For this review, take the finished solid that the model builds, in its own axes (mm). A direction names the side the tool comes from. Give positions to 0.01 mm unless a question says otherwise; leave off trailing zeros. Loops run counter-clockwise (first coordinate to the right, second up) from the corner with the lowest first, then second, coordinate; pieces in that order, holes last.
```python
from build123d import *

# Parameters (mm, degrees)
SKETCH001_W  = 85.039572
SKETCH001_H  = 4.2
POCKET_DEPTH = 20


with BuildPart() as part:
    # CopyCopySketch004 → Revolution (revolve)
    with BuildSketch(Plane.XY):
        with BuildLine():
            Line((-94.301748, 7.336546), (-74.200088, 11.003772))
            ThreePointArc((-66.09792, 11.907295), (-70.164685, 11.596147), (-74.200088, 11.003772))
            Line((-66.09792, 11.907295), (-63.874209, 12))
            Line((-63.874209, 12), (-63.874209, 0))
            Line((-63.874209, 0), (-101.154209, 0))
            ThreePointArc((-94.301748, 7.336546), (-98.941677, 4.801888), (-101.154209, 0))
        make_face()
    revolve(axis=Axis((0, 0, 0), (1, 0, 0)))

    # Sketch001 → Pocket (cut)
    with BuildSketch(Plane.XZ):
        with Locations((-60.179326, 0)):
            Rectangle(SKETCH001_W, SKETCH001_H)
    extrude(amount=-POCKET_DEPTH, mode=Mode.SUBTRACT)


solid = part.part
```
Item 1: For L1, parallel to Y at x = -77, z = -7.5; L2, parallel to Z at x = -96.5, y = 4.25; L3, parallel to Z at x = -98.5, y = 2, list the stretches that pass through material, from the lowest coordinate up.
Answer:
L1: y = -7.34 to 7.34
L2: z = -5.07 to -2.1, 2.1 to 5.07
L3: z = -4.84 to -2.1, 2.1 to 4.84
Item 2: The part is to be moulded in two halves that separate along Z. For faces 3 (the conical face through (-86.34, -8.78, 0.36)), 4 (the flat face through (-83, 0, 0)), 5 (the flat face through (-63.874, -0.3, 0.2)), say which applies: released by +Z, released by -Z, zero draft, split by the parting line, or undercut.
Answer:
face 3: split by the parting line
face 4: undercut
face 5: zero draft
Item 3: Take a section at A-A on x = -84. Give the boundary of the cut face in (y, z).
Answer:
outline: (0, -2.1) - (0, 2.1) - (8.97, 2.1) arc R9.22 ccw (long way) to (8.97, -2.1) - close
Item 4: Clearance check with flat-ended pins moving along their axes: pin 1 Ø2 at (x, z) = (-83, 0) entering from +Y; pin 2 Ø8 at (x, y) = (-95, -9) entering from -Z; pin 3 Ø10 at (x, z) = (-78, 8.5) entering from +Y. State where each tip first meets the part, or that it passes through.
Answer:
pin 1: stops at y = 0
pin 2: stops at z = -5.32
pin 3: stops at y = 9.93
Item 5: Take a section at B-B on x = -76. Give the boundary of the cut face in (y, z).
Answer:
outline: (0, -2.1) - (0, 2.1) - (10.47, 2.1) arc R10.68 ccw (long way) to (10.47, -2.1) - close
Item 6: Tool access review of faces 1 (the conical face through (-65.465, -11.923, 0.495)), 2 (the flat face through (-78, 5, 2.1)): name each direction out of +Z, -Z, +X, -X, +Y, -Y from which nothing blocks a thin tool from reaching the whole face with its end or side.
Answer:
face 1: -X
face 2: +X, -X, +Y
